```python
from build123d import *

# Parameters (mm, degrees)
BOSS_EXTRUDE1_DEPTH    = 9.525
FILLET1_R              = 9.525
FILLET2_R              = 12.7
SKETCH2_R              = 12.7
BOSS_EXTRUDE2_DEPTH    = 63.5
SKETCH4_R              = 12.7
SKETCH4_R_2            = 11.43
CUT_EXTRUDE1_DEPTH     = 0.635
LPATTERN1_COUNT        = 2
LPATTERN1_PITCH        = 21.166666667
SKETCH5_R              = 6.35
BOSS_EXTRUDE3_DEPTH    = 6.35
SKETCH6_R              = 3.81
BOSS_EXTRUDE4_DEPTH    = 2.54
CUT_EXTRUDE2_START     = -1
CUT_EXTRUDE2_OUTLINE_W = 6.477
CUT_EXTRUDE2_OUTLINE_H = 5.588
CUT_EXTRUDE2_DEPTH     = 4.2385
CUT_EXTRUDE2_START_2   = -2.794
CUT_EXTRUDE2_2_DEPTH   = 5.588


with BuildPart() as part:
    # Sketch1 → Boss-Extrude1 (new, symmetric)
    with BuildSketch(Plane(origin=(0, 0, 0), x_dir=(1, 0, 0), z_dir=(0, 1, 0))):
        Polygon((0, -6.35), (0, 6.35), (50.350722524, 6.35), (86.069472524, -50.8), (177.8, -50.8), (177.8, -57.15), (82.55, -57.15), (50.8, -6.35), align=None)
    extrude(amount=BOSS_EXTRUDE1_DEPTH, both=True)

    # Fillet1
    fillet1_edges = [part.edges().sort_by_distance(p)[0] for p in [
        (177.8, -9.525, 53.975),
        (177.8, 9.525, 53.975),
        (0, -9.525, 0),
        (0, 9.525, 0),
    ]]
    fillet(fillet1_edges, radius=FILLET1_R - 0.0001)  # a hair under: the kernel refuses the full size

    # Fillet2
    fillet2_edges = [part.edges().sort_by_distance(p)[0] for p in [
        (50.350722524, 0, -6.35),
        (86.069472524, 0, 50.8),
        (82.55, 0, 57.15),
        (50.8, 0, 6.35),
    ]]
    fillet(fillet2_edges, radius=FILLET2_R)

    # Sketch2 → Boss-Extrude2 (add)
    with BuildSketch(Plane(origin=(0, 0, 50.8), x_dir=(-1, 0, 0), z_dir=(0, 0, -1))):
        with Locations(Location((-168.275, 0, 0), (0, 0, 180))):
            Circle(SKETCH2_R)
    extrude(amount=BOSS_EXTRUDE2_DEPTH)

    # Sketch4 → Cut-Extrude1 (cut, symmetric)
    with BuildSketch(Plane.XY.offset(29.633333333)):
        with Locations((168.275, 0)):
            Circle(SKETCH4_R)
        with Locations((168.275, 0)):
            Circle(SKETCH4_R_2, mode=Mode.SUBTRACT)
    cut_extrude1 = extrude(amount=CUT_EXTRUDE1_DEPTH, both=True, mode=Mode.SUBTRACT)

    # LPattern1: Cut-Extrude1 ×2
    with Locations(*[(0, 0, -i * LPATTERN1_PITCH) for i in range(1, LPATTERN1_COUNT)]):
        add(cut_extrude1, mode=Mode.SUBTRACT)

    # Sketch5 → Boss-Extrude3 (add)
    with BuildSketch(Plane.XY.offset(57.15)):
        with Locations(Location((168.275, 0, 0), (0, 0, 180))):
            Circle(SKETCH5_R)
    extrude(amount=BOSS_EXTRUDE3_DEPTH)

    # Sketch6 → Boss-Extrude4 (add)
    with BuildSketch(Plane.XY.offset(63.5)):
        with Locations((168.275, 0)):
            Circle(SKETCH6_R)
    extrude(amount=BOSS_EXTRUDE4_DEPTH)

    # Cut-Extrude2: read off the stored shape, not the designer's step
    # Cut-Extrude2 outline → Cut-Extrude2 (cut)
    with BuildSketch(Plane.YZ.offset(CUT_EXTRUDE2_START)):
        Rectangle(CUT_EXTRUDE2_OUTLINE_W, CUT_EXTRUDE2_OUTLINE_H)
    extrude(amount=CUT_EXTRUDE2_DEPTH, mode=Mode.SUBTRACT)

    # Cut-Extrude2 2 outline → Cut-Extrude2 2 (cut)
    with BuildSketch(Plane.XY.offset(CUT_EXTRUDE2_START_2)):
        Polygon((9.496069796, -2.159), (9.496069796, 2.159), (3.2385, 3.2385), (3.2385, -3.2385), align=None)
    extrude(amount=CUT_EXTRUDE2_2_DEPTH, mode=Mode.SUBTRACT)


solid = part.part
```
Read the model definition and answer for the solid it produces. Units are mm, in the model's axes. A direction names the side the tool comes from. Coordinates: 2 decimals unless noted, no trailing zeros. Write each loop counter-clockwise with the first axis right and the second up, starting at its lowest first coordinate (ties: lowest second). Pieces come first, ordered by that corner, then holes. Notation, with made-up numbers: (7.25, 84.25) - (20.25, 84.25) arc R15 ccw to (20.25, 95.25) - close; hole circle Ø3 at (78.5, 54). An arc over 180 degrees is marked (long way). Answer as a JSON object with one key per item and string values. Group by question number.
1. A cutting plane is placed at B-B (z = 61). Determine the outline of the cut face in (x, y) (3 decimals).
2. A cutting plane is placed at D-D (x = 48). Determine the outline of the cut face in (y, z) (3 decimals), plus the area to 3 significant figures.
3. Consider L1, parallel to Z at x = 135, y = -1.5; L2, parallel to Z at x = 10, y = 2.5; L3, parallel to X at y = 8.5, z = 44. Determine where each line is inside the solid, lowest interval first. Write a range as [from, to].
4. A cutting plane is placed at C-C (x = 66.5). Determine the outline of the cut face in (y, z) (3 decimals).
5. Each of these flat-tipped pins is pushed along its axis until it touches: P1, Ø15, axis at x = 31.5, y = 3, coming from the -Z side; P2, Ø1, axis at x = 76.5, z = 32, coming from the -Y side; P3, Ø3, axis at x = 117.5, y = -3, coming from the -Z side; P4, Ø6, axis at x = 85, y = -10, coming from the -Z side. Where does it stop, or does it pass through?
6. A cutting plane is placed at A-A (z = 36.5). Determine the outline of the cut face in (x, y) (3 decimals).
7. Which of the six approach directions +Z, -Z, +X, -X, +Y, -Y give full straight-line access (tool end or side, diameter ignored) to faces 1 (the flat face through (22, 0, 6.35)), 2 (the cylindrical face through (175.084, -6.661, 54.019)), 3 (the flat face through (5, 0, -2.794))?
8. The mould has two halves that part along Z. Classify faces 4 (the flat face through (66.845, 0.133, 32.022)), 5 (the flat face through (159, 7, 30.268)), 6 (the cylindrical face through (155.587, -0.558, 19.189)): +Z half, -Z half, draft (parallel to the pull), parting line (faces both ways), or undercut.
Worked out:
{
 "1": {"outline": "circle Ø12.7 at (168.275, 0)"},
 "2": {"outline": "(-9.525, -5.453) - (9.525, -5.453) - (9.525, 7.078) - (-9.525, 7.078) - close", "area": "239 mm²"},
 "3": {"L1": "z = [50.8, 57.15]", "L2": "z = [-6.35, 6.35]", "L3": "x = [74.33, 81.82], [158.84, 177.71]"},
 "4": {"outline": "(-9.525, 19.489) - (9.525, 19.489) - (9.525, 31.47) - (-9.525, 31.47) - close"},
 "5": {"P1": "stops at z = -6.35", "P2": "passes through", "P3": "stops at z = 50.8", "P4": "stops at z = 44.35"},
 "6": {"outline": "(69.644, -9.525) - (77.132, -9.525) - (77.132, 9.525) - (69.644, 9.525) - close; circle Ø25.4 at (168.275, 0)"},
 "7": {"face 1": "+Z, -X, +Y, -Y", "face 2": "+Z, +X, -Y", "face 3": "-X"},
 "8": {"face 4": "+Z half", "face 5": "undercut", "face 6": "draft"}
}
